The model under review builds one solid part; all positions refer to its coordinate system, in mm. A direction names the side the tool comes from. Round coordinates to 2 decimals unless told otherwise and drop trailing zeros. Write each loop counter-clockwise with the first axis right and the second up, starting at its lowest first coordinate (ties: lowest second). Pieces come first, ordered by that corner, then holes. Notation, with made-up numbers: M 39,66 L 92,66 A24 cw 92,90 Z; hole C 11,57 d6. An arc over 180 degrees is marked long. One line per item, written item: value. Start each with the question number.
1) Take a section at A-A, the plane y = 106.5. Write out the cut boundary in (x, z), and give its area (3 significant figures).
2) Take a section at B-B, the plane x = -327. Write out the cut boundary in (y, z).
3) For P1, Ø1, axis at y = 125.5, z = 2.5, coming from the +X side; P2, Ø0.9, axis at y = 131.5, z = 2, coming from the -X side; P3, Ø3, axis at x = -305.76, y = 150.97, coming from the -Z side; P4, Ø1.5, axis at x = -400, z = 2, coming from the -Y side, all flat-tipped, find the tip position at first contact; note any pin that passes through.
4) Wall thickness on probe 1 along Y at (x, z) = (-364, 0.3); probe 2 along X at (y, z) = (150.5, 0.7); probe 3 along Y at (x, z) = (-318, 0.9): over which ranges is each line inside the solid? List them lowest first.
5) Tool access review of faces 5 (the face through (-400, 148.341, 2)), 6 (the face through (-343, 91.188, 2)), 7 (the face through (-314, 111.746, 2)), 8 (the face through (-311, 115.677, 2)): name each direction out of +Z, -Z, +X, -X, +Y, -Y from which nothing blocks a thin tool from reaching the whole face with its end or side.
6) Mouldability with a two-part tool opening along Y and no side actions: class faces 1 (the face through (-401.057, 150, 2)), 2 (the face through (-303, 153.6, 1.5)), 3 (the face through (-399.152, 122, 2)), 4 (the face through (-307.01, 150.45, 1.5)) as +Y half, -Y half, draft (parallel to the pull), parting line (faces both ways), or undercut.
7) Take a section at C-C, the plane z = 2. State how many separate pieces and enclosed holes the cut face has, and give its area (3 significant figures).
from build123d import *

# Parameters (mm, degrees)
BOSS_EXTRUDE1_DEPTH = 3.048
SKETCH2_R           = 1.355900406
CUT_EXTRUDE1_DEPTH  = 430.898988368


with BuildPart() as part:
    # Sketch1 → Boss-Extrude1 (new body)
    with BuildSketch(Plane.XY):
        with BuildLine():
            Line((-309.8086, 128.8851), (-305.87795, 128.8851))
            Line((-305.87795, 128.8851), (-301.9473, 132.81575))
            Line((-301.9473, 132.81575), (-301.9473, 150.9704))
            ThreePointArc((-301.9473, 150.9704), (-303.063223164, 153.664476836), (-305.7573, 154.7804))
            Line((-305.7573, 154.7804), (-397.247125, 154.7804))
            ThreePointArc((-397.247125, 154.7804), (-399.946077222, 153.659592612), (-401.0571, 150.956597849))
            Line((-401.0571, 150.956597849), (-401.0571, 148.341))
            Line((-401.0571, 148.341), (-399.1521, 148.341))
            Line((-399.1521, 148.341), (-399.1521, 95.6449))
            Line((-399.1521, 95.6449), (-401.0571, 95.6449))
            Line((-401.0571, 95.6449), (-401.0571, 91.659304166))
            ThreePointArc((-401.0571, 91.659304166), (-399.951018769, 88.947400452), (-397.2472, 87.8217))
            Line((-397.2472, 87.8217), (-378.5565, 87.8217))
            Line((-378.5565, 87.8217), (-368.3165, 91.1883))
            Line((-368.3165, 91.1883), (-315.9973, 91.1883))
            Line((-315.9973, 91.1883), (-305.7573, 87.8217))
            ThreePointArc((-305.7573, 87.8217), (-303.063223164, 88.937623164), (-301.9473, 91.6317))
            Line((-301.9473, 91.6317), (-301.9473, 111.74645))
            Line((-301.9473, 111.74645), (-305.87795, 115.6771))
            Line((-305.87795, 115.6771), (-309.8086, 115.6771))
            Line((-309.8086, 115.6771), (-316.1078, 115.6771))
            Line((-316.1078, 115.6771), (-316.1078, 128.8851))
            Line((-316.1078, 128.8851), (-309.8086, 128.8851))
        make_face()
        Polygon((-395.3675, 92.9525), (-395.3675, 149.2432), (-309.8086, 149.2432), (-309.8086, 132.81575), (-318.2033, 132.81575), (-318.2033, 111.74645), (-309.8086, 111.74645), (-309.8086, 92.9525), align=None, mode=Mode.SUBTRACT)
    extrude(amount=BOSS_EXTRUDE1_DEPTH)

    # Sketch2 → Cut-Extrude1 (cut, through all)
    with BuildSketch(Plane(origin=(0, 0, 0), x_dir=(-1, 0, 0), z_dir=(0, 0, -1))):
        with Locations((305.7573, 150.9704)):
            Circle(SKETCH2_R)
        with Locations((397.247125, 150.9704)):
            Circle(SKETCH2_R)
        with Locations((397.2472, 91.6317)):
            Circle(SKETCH2_R)
        with Locations((305.7573, 91.6317)):
            Circle(SKETCH2_R)
    extrude(amount=-CUT_EXTRUDE1_DEPTH, mode=Mode.SUBTRACT)


solid = part.part
Checked values:
1. outline: M -399.15,0 L -395.37,0 L -395.37,3.05 L -399.15,3.05 Z; M -309.81,0 L -301.95,0 L -301.95,3.05 L -309.81,3.05 Z
1. area: 35.5 mm2
2. outline: M 91.19,0 L 92.95,0 L 92.95,3.05 L 91.19,3.05 Z; M 149.24,0 L 154.78,0 L 154.78,3.05 L 149.24,3.05 Z
3. P1: stops at x = -316.11
3. P2: stops at x = -399.15
3. P3: stops at z = 0
3. P4: stops at y = 88.39
4. probe 1: y = 91.19 to 92.95, 149.24 to 154.78
4. probe 2: x = -401.06 to -398.52, -395.98 to -307.03, -304.49 to -301.95
4. probe 3: y = 91.19 to 92.95, 111.75 to 132.82, 149.24 to 154.78
5. face 5: +Z, -Z, -X
5. face 6: +Z, -Z, -Y
5. face 7: +Z, -Z
5. face 8: +Z, -Z, +X
6. face 1: draft
6. face 2: +Y half
6. face 3: undercut
6. face 4: undercut
7. separate pieces: 1
7. enclosed holes: 5
7. area: 1,450 mm2
